from build123d import *

# Parameters (mm, degrees)
SKETCH1_R           = 100
SKETCH1_R_2         = 14.75
SKETCH1_R_3         = 25
BOSS_EXTRUDE1_DEPTH = 3
SKETCH1_3_R         = 25
BOSS_EXTRUDE2_DEPTH = 20
SKETCH2_R           = 2.5
BOSS_EXTRUDE3_DEPTH = 1


with BuildPart() as part:
    # Sketch1 → Boss-Extrude1 (new body)
    with BuildSketch(Plane.XY):
        Circle(SKETCH1_R)
        with Locations((80, 0)):
            Circle(SKETCH1_R_2, mode=Mode.SUBTRACT)
        with Locations((71.679501943, -35.525329008)):
            Circle(SKETCH1_R_2, mode=Mode.SUBTRACT)
        with Locations((48.448774971, -63.660947242)):
            Circle(SKETCH1_R_2, mode=Mode.SUBTRACT)
        with Locations((15.140099549, -78.554295781)):
            Circle(SKETCH1_R_2, mode=Mode.SUBTRACT)
        with Locations((-21.317905095, -77.107372685)):
            Circle(SKETCH1_R_2, mode=Mode.SUBTRACT)
        with Locations((-53.341520041, -59.621155974)):
            Circle(SKETCH1_R_2, mode=Mode.SUBTRACT)
        with Locations((-74.269434641, -29.732996453)):
            Circle(SKETCH1_R_2, mode=Mode.SUBTRACT)
        with Locations((-79.748382076, 6.339996549)):
            Circle(SKETCH1_R_2, mode=Mode.SUBTRACT)
        with Locations((-68.638673059, 41.094191326)):
            Circle(SKETCH1_R_2, mode=Mode.SUBTRACT)
        with Locations((-43.251265396, 67.300282626)):
            Circle(SKETCH1_R_2, mode=Mode.SUBTRACT)
        with Locations((-8.867055992, 79.507077157)):
            Circle(SKETCH1_R_2, mode=Mode.SUBTRACT)
        with Locations((27.361611466, 75.175409663)):
            Circle(SKETCH1_R_2, mode=Mode.SUBTRACT)
        Circle(SKETCH1_R_3, mode=Mode.SUBTRACT)
    extrude(amount=BOSS_EXTRUDE1_DEPTH)

    # Sketch1_3 → Boss-Extrude2 (add)
    with BuildSketch(Plane.XY):
        Circle(SKETCH1_3_R)
    extrude(amount=BOSS_EXTRUDE2_DEPTH)

    # Sketch2 → Boss-Extrude3 (add)
    with BuildSketch(Plane.XY.offset(20)):
        Circle(SKETCH2_R)
    extrude(amount=BOSS_EXTRUDE3_DEPTH)


solid = part.part
Work out the finished part from the listing and answer in its coordinate system (mm). A direction names the side the tool comes from. Give positions to 0.01 mm unless a question says otherwise; leave off trailing zeros. Order: outer loops, then holes, each group sorted by start corner. A loop starts at its lowest first (then second) coordinate and runs counter-clockwise, first axis right, second up. Notation, with made-up numbers: M -7,70.5 L 50,70.5 A9 cw 50,75.5 Z; hole C 30,87 d11. An arc over 180 degrees is marked long. Return JSON: item names as keys, results as strings.
Q1. Find section D-D, the plane x = 18. Write down the section's boundary in (y, z), and give its area (3 significant figures).
Answer below:
{"outline": "M -98.37,0 L -93.02,0 L -93.02,3 L -98.37,3 Z; M -64.08,0 L 63.78,0 L 63.78,3 L 17.35,3 L 17.35,20 L -17.35,20 L -17.35,3 L -64.08,3 Z; M 86.57,0 L 98.37,0 L 98.37,3 L 86.57,3 Z", "area": "1,020 mm^2"}
Q2. Find section A-A, the plane y = -85. Write down the section's boundary in (x, z), and give its area (3 significant figures).
Answer below:
{"outline": "M -52.68,0 L -33.78,0 L -33.78,3 L -52.68,3 Z; M -8.86,0 L 1.87,0 L 1.87,3 L -8.86,3 Z; M 28.41,0 L 52.68,0 L 52.68,3 L 28.41,3 Z", "area": "162 mm^2"}
Q3. Find section C-C, the plane y = 50. Write down the section's boundary in (x, z), and give its area (3 significant figures).
Answer below:
{"outline": "M -86.6,0 L -80.4,0 L -80.4,3 L -86.6,3 Z; M -56.88,0 L 86.6,0 L 86.6,3 L -56.88,3 Z", "area": "449 mm^2"}
Q4. Which of the six approach directions +Z, -Z, +X, -X, +Y, -Y give full straight-line access (tool end or side, diameter ignored) to faces 5 (the face through (69.13, 9.97, 1.48)), 6 (the face through (-0.54, -2.44, 20.49))?
Answer below:
{"face 5": "+Z, -Z", "face 6": "+Z"}
Q5. Each of these flat-tipped pins is pushed along its axis until it touches: pin 1 (17.5 mm diameter, centred on x = -74.27, y = -29.73, fed in from +Z) (1 decimal); pin 2 (5 mm diameter, centred on x = 17, y = -19.5, fed in from +Z); pin 3 (8 mm diameter, centred on x = -57.5, y = -3, fed in from -Z). Where does it stop, or does it pass through?
Answer below:
{"pin 1": "passes through", "pin 2": "stops at z = 20", "pin 3": "stops at z = 0"}
Q6. Find section B-B, the plane x = 70.5. Write down the section's boundary in (y, z).
Answer below:
{"outline": "M -70.92,0 L -50.23,0 L -50.23,3 L -70.92,3 Z; M -20.82,0 L -11.28,0 L -11.28,3 L -20.82,3 Z; M 11.28,0 L 70.92,0 L 70.92,3 L 11.28,3 Z"}
Q7. Find the intervals of material crossed by line 1 along X through (y, z) = (13, 2); line 2 along Y through (x, z) = (2, 1.25); line 3 along Z through (x, y) = (-46.5, -74), in increasing order. Write a range as [from, to].
Answer below:
{"line 1": "x = [-99.15, -92.91], [-66.59, 73.03], [86.97, 99.15]", "line 2": "y = [-99.98, -85.26], [-71.85, 69.53], [89.48, 99.98]", "line 3": "z = [0, 3]"}
Q8. The mould has two halves that part along X. Classify faces 1 (the face through (-45.171, 81.925, 1.479)), 2 (the face through (0, -5, 20)), 3 (the face through (23.846, 7.509, 11.381)), 4 (the face through (-46.54, -72.71, 1.48)): pulls with the +X half, pulls with the -X half, needs draft (parallel to the pull), parting line crosses it, or undercut.
Answer below:
{"face 1": "undercut", "face 2": "needs draft", "face 3": "parting line crosses it", "face 4": "undercut"}
